Answer from the drawing. Dimensions are ordinates in mm from the lowest x, y and z of the part. A direction names the side the tool comes from. Coordinates: 2 decimals unless noted, no trailing zeros. Write each loop counter-clockwise with the first axis right and the second up, starting at its lowest first coordinate (ties: lowest second). Pieces come first, ordered by that corner, then holes. Notation, with made-up numbers: (64.25, -31.5) - (76.25, -31.5) arc R24 cw to (76.25, -12.5) - close; hole circle Ø7 at (-6, -31.75). An arc over 180 degrees is marked (long way). Use one line per item in the form item = value. Start each with the question number.
Item 1: Consider probe 1 along Z at (x, y) = (146, 2); probe 2 along X at (y, z) = (42, 43); probe 3 along Y at (x, z) = (151.5, 32.5). Determine where each line is inside the solid, lowest interval first.
Item 2: Given pin 1 (3.5 mm diameter, centred on y = 1, z = 17, fed in from -X); pin 2 (9 mm diameter, centred on x = 143.5, z = 33.5, fed in from -Y); pin 3 (13.5 mm diameter, centred on x = 146, z = 11.5, fed in from -Y); pin 4 (3 mm diameter, centred on x = 161, z = 6, fed in from +Y), each flat-ended and moving along its own axis, determine where each tip first touches the part or whether it passes through.
Item 3: Determine the mould class of the marked faces 3, 4, 5 and 6 for opening direction X: released by +X, released by -X, zero draft, split by the parting line, or undercut.
Item 4: For the marked faces 1 and 2, determine the directions among +Z, -Z, +X, -X, +Y, -Y from which every point of the face is accessible in a straight line to the end or side of a thin tool.
Item 5: A cutting plane is placed at D-D (z = 51). Write down the section's boundary in (x, y), then the cut area to 3 significant figures.
Item 6: A cutting plane is placed at A-A (z = 11.5). Give the number of separate pieces and of enclosed holes in the cut face, then the cut area to 3 significant figures.
Item 7: A cutting plane is placed at C-C (y = 42.5). Write down the section's boundary in (x, z).
Item 8: A cutting plane is placed at B-B (x = 100). Write down the section's boundary in (y, z), then the cut area to 3 significant figures.
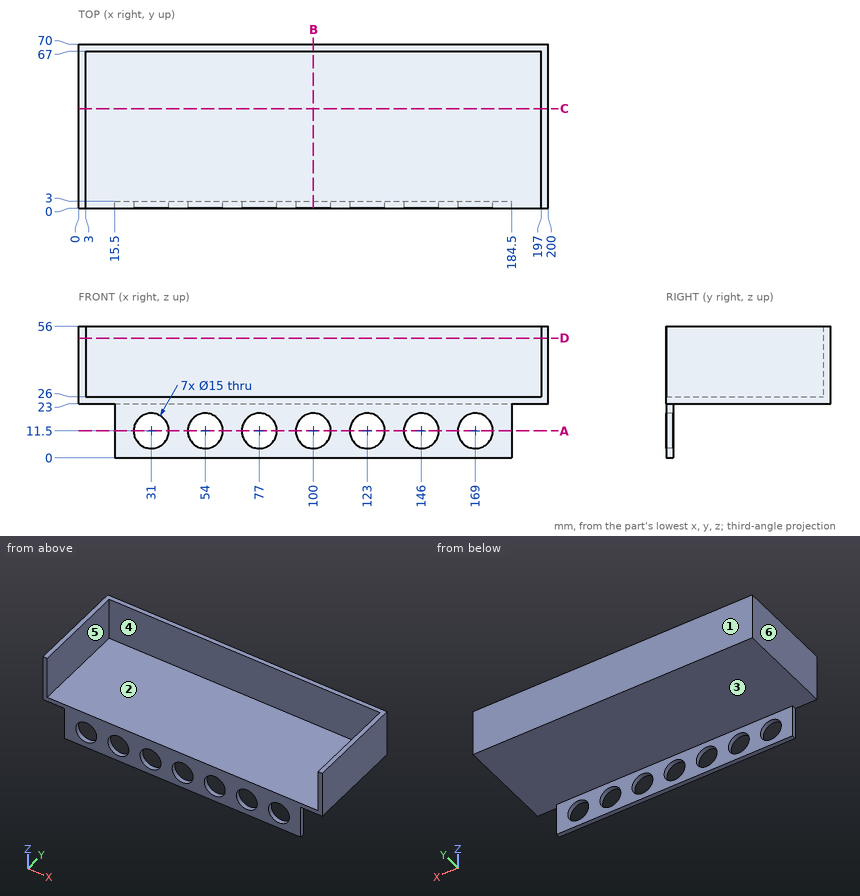
Answer:
q1.probe_1 = 0 to 4, 19 to 26
q1.probe_2 = 0 to 3, 197 to 200
q1.probe_3 = 67 to 70
q2.pin_1 = 15.5
q2.pin_2 = 67
q2.pin_3 = through
q2.pin_4 = 3
q3.face_3 = zero draft
q3.face_4 = undercut
q3.face_5 = undercut
q3.face_6 = released by -X
q4.face_1 = +Z, -Z, +X, -X, +Y
q4.face_2 = +Z, -Y
q5.outline = (0, 0) - (3, 0) - (3, 67) - (197, 67) - (197, 0) - (200, 0) - (200, 70) - (0, 70) - close
q5.area = 1,000 mm²
q6.separate_pieces = 8
q6.enclosed_holes = 0
q6.area = 192 mm²
q7.outline = (0, 23) - (200, 23) - (200, 56) - (197, 56) - (197, 26) - (3, 26) - (3, 56) - (0, 56) - close
q8.outline = (0, 0) - (3, 0) - (3, 4) - (0, 4) - close; (0, 19) - (3, 19) - (3, 23) - (70, 23) - (70, 56) - (67, 56) - (67, 26) - (0, 26) - close
q8.area = 324 mm²
